Could you check a few things on this model? Use its own coordinates, in mm. A direction names the side the tool comes from. Give positions to 0.01 mm unless a question says otherwise; leave off trailing zeros. Write each loop counter-clockwise with the first axis right and the second up, starting at its lowest first coordinate (ties: lowest second). Pieces come first, ordered by that corner, then holes. Notation, with made-up numbers: (81.25, 35) - (120.25, 35) arc R22 ccw to (120.25, 64) - close; hole circle Ø4 at (12, 59). An arc over 180 degrees is marked (long way). Answer as CSV lines item,"result". Start each with the question number.
Q1. Imagine slicing it at C-C on z = -6. List the corners of the cut face in (x, y) for me (3 decimals), and give its area (3 significant figures).
Q2. Imagine slicing it at D-D on y = 132.08. List the corners of the cut face in (x, z) for me (3 decimals), and give its area (3 significant figures).
Q3. If I drill on line 1 along Y through (x, z) = (-16, -6.5); line 2 along X through (y, z) = (132.08, -22.9); line 3 along Z through (x, y) = (-9.5, 111), over which ranges is the centre line in solid material (lowest first)?
Q4. Imagine slicing it at A-A on y = 101.6. State how many separate pieces and enclosed holes the cut face has, and give its area (3 significant figures).
Q5. We'd pull the mould along Z, two halves only. Please class faces 5 (the face through (17.485, 66.405, 17.905)), 6 (the face through (-13.08, 74.49, -22.06)): pulls with the +Z half, pulls with the -Z half, needs draft (parallel to the pull), parting line crosses it, or undercut.
Q6. Will these pins go through, and if not, where does the flat tip stop? pin 1 Ø6 at (x, z) = (1, 15.5) entering from +Y; pin 2 Ø12 at (x, z) = (6.5, 15.5) entering from -Y.
Q7. Imagine slicing it at B-B on x = 3.5. List the corners of the cut face in (y, z) for me, and give its area (3 significant figures).
Q8. On a 3-axis mill with a long thin cutter (end or side, diameter ignored), from which of +Z, -Z, +X, -X, +Y, -Y can I reach the whole of each face in a straight line? I mean faces 1 (the face through (17.48, 42.86, 17.95)), 2 (the face through (-17.48, 126.46, -16.95)), 3 (the face through (13.84, 130.37, -22.06)), 4 (the face through (-15.875, 76, -1)). Say none if no direction works.
```python
from build123d import *

# Parameters (mm, degrees)
SKETCH1_W               = 38.1
SKETCH1_H               = 47.244
SKETCH1_W_2             = 31.75
SKETCH1_H_2             = 40.894
BOSS_EXTRUDE1_DEPTH     = 152.4
SKETCH2_R               = 1.89865
CUT_EXTRUDE1_DEPTH      = 35.925
CUT_EXTRUDE1_DEPTH_BACK = 4.175
CUT_EXTRUDE3_DEPTH      = 3.175
CUT_EXTRUDE4_DEPTH      = 3.175
SKETCH6_R               = 9.525
SKETCH6_R_2             = 2.5527
CUT_EXTRUDE5_DEPTH      = 3.175
CUT_EXTRUDE6_DEPTH      = 3.175
F_6_32_TAPPED_HOLE1_D   = 3.5052
CUT_EXTRUDE10_REACH     = 49.244
SKETCH15_R              = 1.7526


with BuildPart() as part:
    # Sketch1 → Boss-Extrude1 (new body)
    with BuildSketch(Plane(origin=(0, 0, 0), x_dir=(1, 0, 0), z_dir=(0, 1, 0))):
        Rectangle(SKETCH1_W, SKETCH1_H)
        Rectangle(SKETCH1_W_2, SKETCH1_H_2, mode=Mode.SUBTRACT)
    extrude(amount=BOSS_EXTRUDE1_DEPTH)

    # Sketch2 → Cut-Extrude1 (cut, two sides)
    with BuildSketch(Plane.ZY.offset(-15.875)) as cut_extrude1_sk:
        with Locations((-16.645384182, 6.21538)):
            Circle(SKETCH2_R)
        with Locations((10.30030417, 6.18241423)):
            Circle(SKETCH2_R)
    extrude(amount=CUT_EXTRUDE1_DEPTH, mode=Mode.SUBTRACT)
    extrude(cut_extrude1_sk.sketch, amount=-CUT_EXTRUDE1_DEPTH_BACK, mode=Mode.SUBTRACT)

    # Sketch4 → Cut-Extrude3 (cut)
    with BuildSketch(Plane.ZY.offset(19.05)):
        with BuildLine():
            Line((15.6845, 10.16), (-15.6845, 10.16))
            ThreePointArc((-15.6845, 10.16), (-17.92956403, 11.08993597), (-18.8595, 13.335))
            Line((-18.8595, 13.335), (-18.8595, 64.135))
            ThreePointArc((-18.8595, 64.135), (-17.92956403, 66.38006403), (-15.6845, 67.31))
            Line((-15.6845, 67.31), (15.6845, 67.31))
            ThreePointArc((15.6845, 67.31), (17.92956403, 66.38006403), (18.8595, 64.135))
            Line((18.8595, 64.135), (18.8595, 13.335))
            ThreePointArc((18.8595, 13.335), (17.92956403, 11.08993597), (15.6845, 10.16))
        make_face()
    extrude(amount=-CUT_EXTRUDE3_DEPTH, mode=Mode.SUBTRACT)

    # Sketch5 → Cut-Extrude4 (cut)
    with BuildSketch(Plane(origin=(19.05, 0, 0), x_dir=(0, 0, -1), z_dir=(1, 0, 0))):
        with BuildLine():
            Line((15.6845, 67.31), (-15.6845, 67.31))
            ThreePointArc((-15.6845, 67.31), (-17.92956403, 66.38006403), (-18.8595, 64.135))
            Line((-18.8595, 64.135), (-18.8595, 45.085))
            ThreePointArc((-18.8595, 45.085), (-17.92956403, 42.83993597), (-15.6845, 41.91))
            Line((-15.6845, 41.91), (15.6845, 41.91))
            ThreePointArc((15.6845, 41.91), (17.92956403, 42.83993597), (18.8595, 45.085))
            Line((18.8595, 45.085), (18.8595, 64.135))
            ThreePointArc((18.8595, 64.135), (17.92956403, 66.38006403), (15.6845, 67.31))
        make_face()
    extrude(amount=-CUT_EXTRUDE4_DEPTH, mode=Mode.SUBTRACT)

    # Sketch6 → Cut-Extrude5 (cut)
    with BuildSketch(Plane.ZY.offset(-15.875)):
        with Locations((0, 101.6)):
            Circle(SKETCH6_R)
        with Locations((0, 87.63)):
            Circle(SKETCH6_R_2)
        with Locations((-9.878281733, 91.721718267)):
            Circle(SKETCH6_R_2)
        with Locations((-13.97, 101.6)):
            Circle(SKETCH6_R_2)
        with Locations((-9.878281733, 111.478281733)):
            Circle(SKETCH6_R_2)
        with Locations((0, 115.57)):
            Circle(SKETCH6_R_2)
        with Locations((9.878281733, 111.478281733)):
            Circle(SKETCH6_R_2)
        with Locations((13.97, 101.6)):
            Circle(SKETCH6_R_2)
        with Locations((9.878281733, 91.721718267)):
            Circle(SKETCH6_R_2)
    extrude(amount=-CUT_EXTRUDE5_DEPTH, mode=Mode.SUBTRACT)

    # Sketch7 → Cut-Extrude6 (cut)
    with BuildSketch(Plane.ZY.offset(19.05)):
        with BuildLine():
            Line((-12.5095, 77.47), (12.5095, 77.47))
            ThreePointArc((12.5095, 77.47), (16.999628061, 79.329871939), (18.8595, 83.82))
            Line((18.8595, 83.82), (18.8595, 121.92))
            ThreePointArc((18.8595, 121.92), (16.999628061, 126.410128061), (12.5095, 128.27))
            Line((12.5095, 128.27), (-12.5095, 128.27))
            ThreePointArc((-12.5095, 128.27), (-16.999628061, 126.410128061), (-18.8595, 121.92))
            Line((-18.8595, 121.92), (-18.8595, 83.82))
            ThreePointArc((-18.8595, 83.82), (-16.999628061, 79.329871939), (-12.5095, 77.47))
        make_face()
    extrude(amount=-CUT_EXTRUDE6_DEPTH, mode=Mode.SUBTRACT)

    # #6-32 Tapped Hole1 (through all)
    with Locations(Plane(origin=(19.05, 73.406, -13.423592181), x_dir=(0, 0, 1), z_dir=(1, 0, 0))):
        with Locations((0, 0), (26.924, 0), (26.924, -72.644), (0, -72.644)):
            Hole(F_6_32_TAPPED_HOLE1_D / 2)

    # Sketch15 → Cut-Extrude10 (cut, up to next)
    with BuildSketch(Plane(origin=(0, 0, -23.622), x_dir=(-1, 0, 0), z_dir=(0, 0, -1)), mode=Mode.PRIVATE) as cut_extrude10_sk1:
        with Locations((-13.462, 50.8)):
            Circle(SKETCH15_R)
    cut_extrude10_tool1 = extrude(cut_extrude10_sk1.sketch, amount=-CUT_EXTRUDE10_REACH, mode=Mode.PRIVATE) & part.part
    add(cut_extrude10_tool1.solids().sort_by_distance((13.462, 50.8, -23.622))[0], mode=Mode.SUBTRACT)
    # Sketch15 → Cut-Extrude10 (cut, up to next)
    with BuildSketch(Plane(origin=(0, 0, -23.622), x_dir=(-1, 0, 0), z_dir=(0, 0, -1)), mode=Mode.PRIVATE) as cut_extrude10_sk2:
        with Locations((13.462, 50.8)):
            Circle(SKETCH15_R)
    cut_extrude10_tool2 = extrude(cut_extrude10_sk2.sketch, amount=-CUT_EXTRUDE10_REACH, mode=Mode.PRIVATE) & part.part
    add(cut_extrude10_tool2.solids().sort_by_distance((-13.462, 50.8, -23.622))[0], mode=Mode.SUBTRACT)
    # Sketch15 → Cut-Extrude10 (cut, up to next)
    with BuildSketch(Plane(origin=(0, 0, -23.622), x_dir=(-1, 0, 0), z_dir=(0, 0, -1)), mode=Mode.PRIVATE) as cut_extrude10_sk3:
        with Locations((-13.462, 76.2)):
            Circle(SKETCH15_R)
    cut_extrude10_tool3 = extrude(cut_extrude10_sk3.sketch, amount=-CUT_EXTRUDE10_REACH, mode=Mode.PRIVATE) & part.part
    add(cut_extrude10_tool3.solids().sort_by_distance((13.462, 76.2, -23.622))[0], mode=Mode.SUBTRACT)
    # Sketch15 → Cut-Extrude10 (cut, up to next)
    with BuildSketch(Plane(origin=(0, 0, -23.622), x_dir=(-1, 0, 0), z_dir=(0, 0, -1)), mode=Mode.PRIVATE) as cut_extrude10_sk4:
        with Locations((13.462, 76.2)):
            Circle(SKETCH15_R)
    cut_extrude10_tool4 = extrude(cut_extrude10_sk4.sketch, amount=-CUT_EXTRUDE10_REACH, mode=Mode.PRIVATE) & part.part
    add(cut_extrude10_tool4.solids().sort_by_distance((-13.462, 76.2, -23.622))[0], mode=Mode.SUBTRACT)
    # Sketch15 → Cut-Extrude10 (cut, up to next)
    with BuildSketch(Plane(origin=(0, 0, -23.622), x_dir=(-1, 0, 0), z_dir=(0, 0, -1)), mode=Mode.PRIVATE) as cut_extrude10_sk5:
        with Locations((-13.462, 132.08)):
            Circle(SKETCH15_R)
    cut_extrude10_tool5 = extrude(cut_extrude10_sk5.sketch, amount=-CUT_EXTRUDE10_REACH, mode=Mode.PRIVATE) & part.part
    add(cut_extrude10_tool5.solids().sort_by_distance((13.462, 132.08, -23.622))[0], mode=Mode.SUBTRACT)
    # Sketch15 → Cut-Extrude10 (cut, up to next)
    with BuildSketch(Plane(origin=(0, 0, -23.622), x_dir=(-1, 0, 0), z_dir=(0, 0, -1)), mode=Mode.PRIVATE) as cut_extrude10_sk6:
        with Locations((13.462, 132.08)):
            Circle(SKETCH15_R)
    cut_extrude10_tool6 = extrude(cut_extrude10_sk6.sketch, amount=-CUT_EXTRUDE10_REACH, mode=Mode.PRIVATE) & part.part
    add(cut_extrude10_tool6.solids().sort_by_distance((-13.462, 132.08, -23.622))[0], mode=Mode.SUBTRACT)


solid = part.part
```
Conclusion:
1,outline,"(-19.05, 0) - (-15.875, 0) - (-15.875, 10.16) - (-19.05, 10.16) - close; (-19.05, 67.31) - (-15.875, 67.31) - (-15.875, 77.47) - (-19.05, 77.47) - close; (-19.05, 128.27) - (-15.875, 128.27) - (-15.875, 152.4) - (-19.05, 152.4) - close; (15.875, 0) - (19.05, 0) - (19.05, 41.91) - (15.875, 41.91) - close; (15.875, 67.31) - (19.05, 67.31) - (19.05, 94.202) - (15.875, 94.202) - close; (15.875, 108.998) - (19.05, 108.998) - (19.05, 152.4) - (15.875, 152.4) - close"
1,area,"497 mm^2"
2,outline,"(-19.05, -23.622) - (-15.215, -23.622) - (-15.215, -20.447) - (-15.875, -20.447) - (-15.875, 20.447) - (15.875, 20.447) - (15.875, -20.447) - (15.215, -20.447) - (15.215, -23.622) - (19.05, -23.622) - (19.05, 23.622) - (-19.05, 23.622) - close; (-11.709, -23.622) - (11.709, -23.622) - (11.709, -20.447) - (-11.709, -20.447) - close"
2,area,"479 mm^2"
3,line 1,"0 to 10.16, 67.31 to 77.47, 128.27 to 152.4"
3,line 2,"-19.05 to -15.21, -11.71 to 11.71, 15.21 to 19.05"
3,line 3,"-23.62 to -20.45, 20.45 to 23.62"
4,separate pieces,"4"
4,enclosed holes,"0"
4,area,"289 mm^2"
5,face 5,"undercut"
5,face 6,"needs draft"
6,pin 1,"through"
6,pin 2,"y = 0"
7,outline,"(0, -23.62) - (152.4, -23.62) - (152.4, -20.45) - (0, -20.45) - close; (0, 20.45) - (152.4, 20.45) - (152.4, 23.62) - (0, 23.62) - close"
7,area,"968 mm^2"
8,face 1,"+X, -X"
8,face 2,"-X"
8,face 3,"-Z"
8,face 4,"+Y, -Y"
